from build123d import *

# Parameters (mm, degrees)
SKETCH_W     = 30
SKETCH_H     = 80
SKETCH_R     = 2.5
PAD_DEPTH    = 5
SKETCH001_R  = 2.5
PAD001_DEPTH = 3
SKETCH002_R  = 1.1
POCKET_DEPTH = 5
FILLET_R     = 6


with BuildPart() as part:
    # Sketch → Pad (new body)
    with BuildSketch(Plane.XY):
        with Locations((15, 40)):
            Rectangle(SKETCH_W, SKETCH_H)
        with Locations((25, 4)):
            Circle(SKETCH_R, mode=Mode.SUBTRACT)
        with Locations((25, 75)):
            Circle(SKETCH_R, mode=Mode.SUBTRACT)
    extrude(amount=PAD_DEPTH)

    # Sketch001 (on Face8 of Pad) → Pad001 (join)
    with BuildSketch(Plane.XY.offset(5)):
        with Locations((2.54, 6.6)):
            Circle(SKETCH001_R)
        with Locations((18.542, 36.58)):
            Circle(SKETCH001_R)
    extrude(amount=PAD001_DEPTH)

    # Sketch002 (on DatumPlane) → Pocket (cut)
    with BuildSketch(Plane.XY.offset(8)):
        with Locations((2.583942, 6.530214)):
            Circle(SKETCH002_R)
        with Locations((18.499644, 36.530405)):
            Circle(SKETCH002_R)
    extrude(amount=-POCKET_DEPTH, mode=Mode.SUBTRACT)

    # Fillet
    fillet_edges = [part.edges().sort_by_distance(p)[0] for p in [
        (30, 0, 2.5),
        (0, 0, 2.5),
        (30, 80, 2.5),
        (0, 80, 2.5),
    ]]
    fillet(fillet_edges, radius=FILLET_R)


solid = part.part
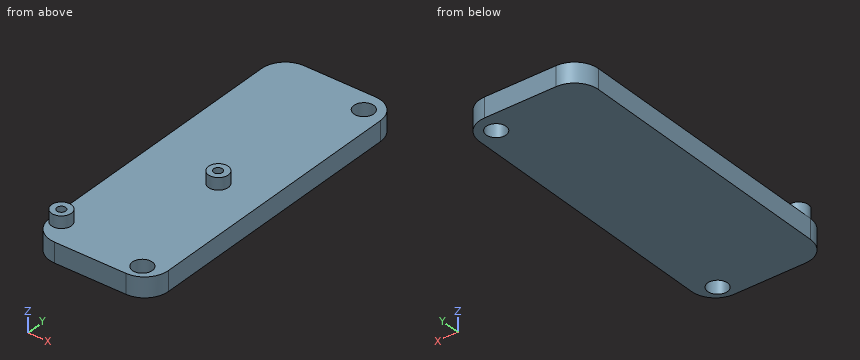
Design review of the part built by this model. Coordinates are the model's own, in mm. Coordinates: 2 decimals unless noted, no trailing zeros. Loops run counter-clockwise (first coordinate to the right, second up) from the corner with the lowest first, then second, coordinate; pieces in that order, holes last.
Item 1: Add section C-C (x = 2.54). Write out the cut boundary in (y, z).
Completed:
outline: (1.1, 0) - (78.9, 0) - (78.9, 5) - (9.1, 5) - (9.1, 8) - (7.63, 8) - (7.63, 3) - (5.43, 3) - (5.43, 8) - (4.1, 8) - (4.1, 5) - (1.1, 5) - close
Item 2: Wall thickness on L1, parallel to Y at x = 25, z = 3.55; L2, parallel to Z at x = 20.5, y = 52; L3, parallel to Y at x = 18, z = 7: over which ranges is each line inside the solid? List them lowest first.
Completed:
L1: y = 0.08 to 1.5, 6.5 to 72.5, 77.5 to 79.92
L2: z = 0 to 5
L3: y = 34.14 to 35.55, 37.51 to 39.02
Item 3: Add section D-D (z = 6.25). Write out the cut boundary in (x, y), and give its area (3 significant figures).
Completed:
outline: circle Ø5 at (2.54, 6.6); circle Ø5 at (18.54, 36.58); hole circle Ø2.2 at (2.58, 6.53); hole circle Ø2.2 at (18.5, 36.53)
area: 31.7 mm2
Item 4: Add section A-A (z = 2). Write out the cut boundary in (x, y).
Completed:
outline: (0, 6) arc R6 ccw to (6, 0) - (24, 0) arc R6 ccw to (30, 6) - (30, 74) arc R6 ccw to (24, 80) - (6, 80) arc R6 ccw to (0, 74) - close; hole circle Ø5 at (25, 4); hole circle Ø5 at (25, 75)
Item 5: Clearance check with flat-ended pins moving along their axes: pin 1 (8 mm diameter, centred on x = 13.5, y = 64.5, fed in from +Z); pin 2 (3 mm diameter, centred on x = 25, y = 4, fed in from -Z); pin 3 (2 mm diameter, centred on x = 18.5, y = 36.53, fed in from +Z). State where each tip first meets the part, or that it passes through.
Completed:
pin 1: stops at z = 5
pin 2: passes through
pin 3: stops at z = 3
Item 6: Add section B-B (x = 25). Write out the cut boundary in (y, z), and give its area (3 significant figures).
Completed:
outline: (0.08, 0) - (1.5, 0) - (1.5, 5) - (0.08, 5) - close; (6.5, 0) - (72.5, 0) - (72.5, 5) - (6.5, 5) - close; (77.5, 0) - (79.92, 0) - (79.92, 5) - (77.5, 5) - close
area: 349 mm2
